Source: three-view drawing plus pictorial views. Frame: mm from the lowest corner of the part. Round coordinates to 2 decimals unless told otherwise and drop trailing zeros. Order: outer loops, then holes, each group sorted by start corner. A loop starts at its lowest first (then second) coordinate and runs counter-clockwise, first axis right, second up. Notation, with made-up numbers: (-38, -30.75) - (21, -30.75) arc R23 ccw to (21, -22.75) - close; hole circle Ø11 at (10.5, 78.5). An arc over 180 degrees is marked (long way). Use one line per item in the form item = value. Start each with the question number.
Q1. Cut plane C-C, the plane z = 23. Return the cut outline in (x, y) (1 decimal).
Q2. Cut plane A-A, the plane x = 19.5. Return the cut outline in (y, z) (1 decimal).
Q3. Pin query (flat end, axial travel): pin 1 Ø5 at (x, z) = (42.5, 10.5) entering from -Y; pin 2 Ø3 at (x, z) = (54, 28) entering from +Y. Return the tip coordinate at first contact, or that it passes through.
Q4. Cut plane B-B, the plane y = 35. Return the cut outline in (x, z) (1 decimal).
Q5. Ray query, line 1 (Z direction, x = 81.5, y = 23.5); line 2 (Y direction, x = 37, z = 28.5) (1 decimal); line 3 (Z direction, x = 9.5, y = 257.5). Return the intervals inside material, ascending. Write a range as [from, to].
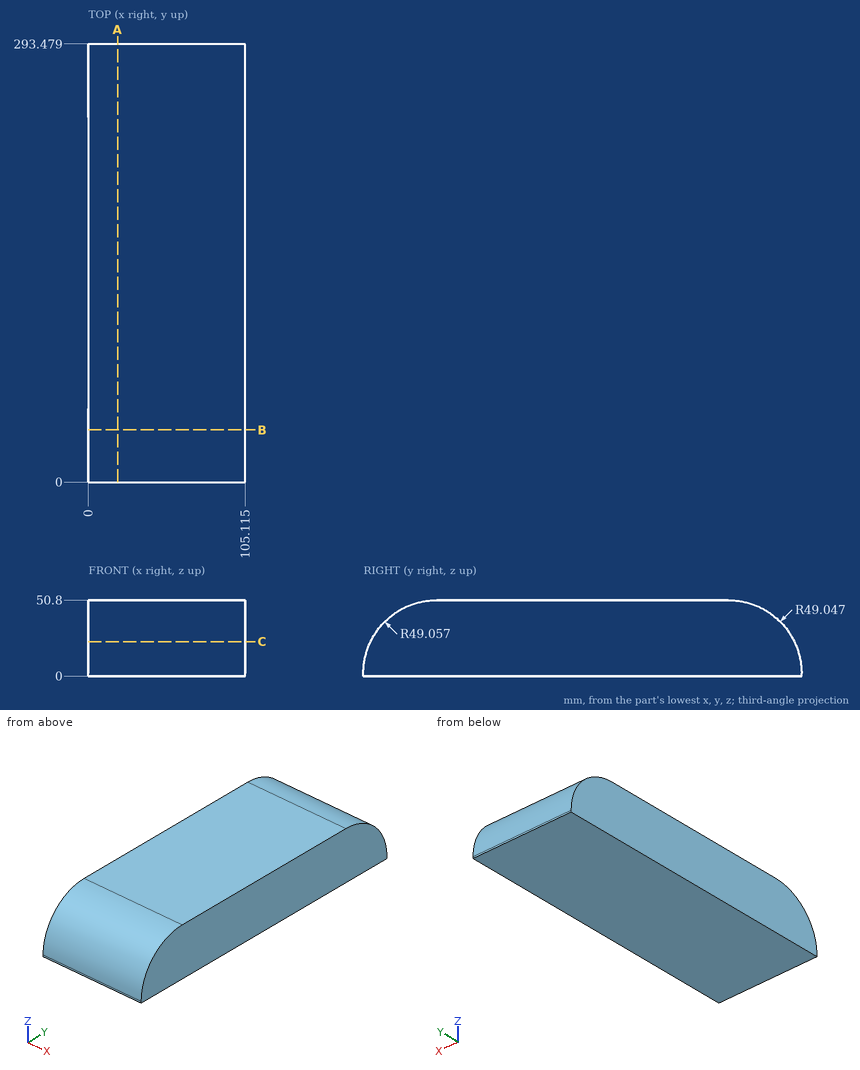
Completed:
q1.outline = (0, 4.8) - (105.1, 4.8) - (105.1, 288.6) - (0, 288.6) - close
q2.outline = (0, 0) - (293.5, 0) - (293.5, 1.8) arc R49 ccw to (244.4, 50.8) - (49.1, 50.8) arc R49.1 ccw to (0, 1.7) - close
q3.pin_1 = 0.4
q3.pin_2 = 286.78
q4.outline = (0, 0) - (105.1, 0) - (105.1, 48.7) - (0, 48.7) - close
q5.line_1 = [0, 43.62]
q5.line_2 = [7.9, 285.5]
q5.line_3 = [0, 49.03]
